Can you work these out from the drawing? Everything is in mm from the part's minimum corner. Give positions to 0.01 mm unless a question says otherwise; leave off trailing zeros. Loops run counter-clockwise (first coordinate to the right, second up) from the corner with the lowest first, then second, coordinate; pieces in that order, holes last. Notation, with made-up numbers: (73.5, -38) - (126.5, -38) arc R20 ccw to (126.5, -18) - close; hole circle Ø5 at (52, -21.5). An arc over 180 degrees is marked (long way). Answer in a Markdown table with one row per item.
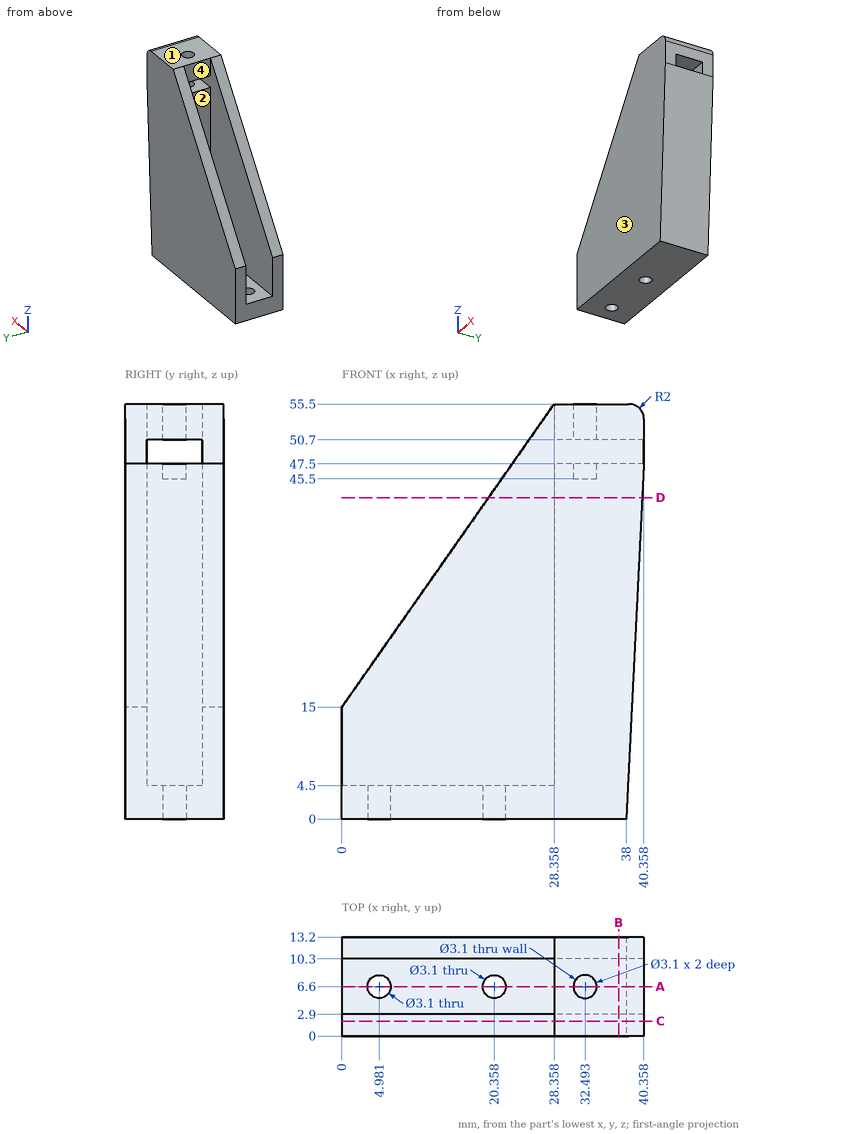
Q1. Imagine slicing it at A-A, the plane y = 6.6. Write out the boundary of the cut face in (x, z).
Checked values:
| item | result |
|---|---|
| outline | (0, 0) - (3.43, 0) - (3.43, 4.5) - (0, 4.5) - close; (6.53, 0) - (18.81, 0) - (18.81, 4.5) - (6.53, 4.5) - close; (21.91, 0) - (38, 0) - (40.36, 47.5) - (34.04, 47.5) - (34.04, 45.5) - (30.94, 45.5) - (30.94, 47.5) - (28.36, 47.5) - (28.36, 4.5) - (21.91, 4.5) - close; (28.36, 50.7) - (30.94, 50.7) - (30.94, 55.5) - (28.36, 55.5) - close; (34.04, 50.7) - (40.36, 50.7) - (40.36, 53.5) arc R2 ccw to (38.36, 55.5) - (34.04, 55.5) - close |
Q2. If we mould it in two halves opening along Y, with no side actions, what happens to the marked faces 1, 2, 3 and 4? For each: released by +Y, released by -Y, zero draft, split by the parting line, or undercut.
Checked values:
| item | result |
|---|---|
| face 1 | zero draft |
| face 2 | undercut |
| face 3 | released by -Y |
| face 4 | undercut |
Q3. Imagine slicing it at C-C, the plane y = 2. Write out the boundary of the cut face in (x, z).
Checked values:
| item | result |
|---|---|
| outline | (0, 0) - (38, 0) - (40.36, 47.5) - (40.36, 53.5) arc R2 ccw to (38.36, 55.5) - (28.36, 55.5) - (0, 15) - close |
Q4. Imagine slicing it at D-D, the plane z = 43. Write out the boundary of the cut face in (x, y) (1 decimal).
Checked values:
| item | result |
|---|---|
| outline | (19.6, 0) - (40.1, 0) - (40.1, 13.2) - (19.6, 13.2) - (19.6, 10.3) - (28.4, 10.3) - (28.4, 2.9) - (19.6, 2.9) - close |
Q5. If I drill on line 1 (Y direction, x = 25.5, z = 49.5); line 2 (X direction, y = 6.6, z = 3.3); line 3 (Z direction, x = 33, y = 9), over which ranges is the centre line in solid material (lowest first)? Write a range as [from, to].
Checked values:
| item | result |
|---|---|
| line 1 | y = [0, 2.9], [10.3, 13.2] |
| line 2 | x = [0, 3.43], [6.53, 18.81], [21.91, 38.16] |
| line 3 | z = [0, 47.5], [50.7, 55.5] |
Q6. Imagine slicing it at B-B, the plane x = 37. Write out the boundary of the cut face in (y, z), and give its area (3 significant figures).
Checked values:
| item | result |
|---|---|
| outline | (0, 0) - (13.2, 0) - (13.2, 55.5) - (0, 55.5) - close; hole (2.9, 47.5) - (10.3, 47.5) - (10.3, 50.7) - (2.9, 50.7) - close |
| area | 709 mm² |
Q7. For pin 1 (1.5 mm diameter, centred on x = 14.5, y = 4, fed in from +Z); pin 2 (4 mm diameter, centred on y = 7.5, z = 52, fed in from -X); pin 3 (6 mm diameter, centred on y = 8, z = 21.5, fed in from -X), each with a flat end and sliding along its axis, tell me the tip position at first contact or that it passes through.
Checked values:
| item | result |
|---|---|
| pin 1 | stops at z = 4.5 |
| pin 2 | stops at x = 28.36 |
| pin 3 | stops at x = 3.2 |
